Input: part model. Units: mm. Frame: model coordinates. A direction names the side the tool comes from. Round coordinates to 2 decimals unless told otherwise and drop trailing zeros. Order: outer loops, then holes, each group sorted by start corner. A loop starts at its lowest first (then second) coordinate and runs counter-clockwise, first axis right, second up. Notation, with made-up numbers: (65, -15) -> (104, -15) arc R20 cw to (104, -3) -> close; hole circle Ø10 at (-20, -9). An arc over 180 degrees is marked (long way). Answer as CSV lines item,"result". Start each with the question number.
1) Line query: L1, parallel to X at y = -3.75, z = 5.05; L2, parallel to Y at x = 6, z = 2.6; L3, parallel to X at y = 4, z = 2.95. Output: solid intervals per line, ascending.
2) Section query A-A, the plane z = 3.7. Output: boundary loops of the cut face in (x, y), and give its area (3 significant figures).
3) First-contact query: P1, Ø1.8, axis at x = 10, y = -5, coming from the +Z side; P2, Ø0.8, axis at x = 16, y = -3, coming from the +Z side; P3, Ø3, axis at x = 6.5, y = 2.5, coming from the +Z side. Flat tips, straight axial feed; report the tip coordinate or a pass-through.
4) Access query for faces 1 (the face through (1, -5, 5.3)), 2 (the face through (0.5, 1.9, 1.9)), 3 (the face through (16, 3.95, 5)), 4 (the face through (8, 4.25, 4)), 5 (the face through (0.5, 3.95, 4.5)). Directions: +Z, -Z, +X, -X, +Y, -Y. A direction counts if a zero-diameter tool reaches every point of the face in a straight line with its end or side. Return the directions, or none.
5) Section query C-C, the plane y = -1.5. Output: boundary loops of the cut face in (x, z), and give its area (3 significant figures).
6) Section query D-D, the plane z = 2.6. Output: boundary loops of the cut face in (x, y).
7) Mould query, pull axis X, two halves, no side actions, for faces 6 (the face through (2, 0, 4)), 7 (the face through (16.5, 4.3, 2.9)), 8 (the face through (16, 3, 2.9)). Classes: +X half, -X half, draft (parallel to the pull), parting line (faces both ways), or undercut.
8) Section query B-B, the plane x = 2.8. Output: boundary loops of the cut face in (y, z), and give its area (3 significant figures).
```python
from build123d import *

# Parameters (mm, degrees)
BOX019_W          = 12.3
BOX019_H          = 9.7
BOX019_DEPTH      = 1
CYLINDER004_R     = 0.8
CYLINDER004_DEPTH = 20
BOX018_W          = 1.6
BOX018_H          = 20
BOX018_DEPTH      = 3
BOX017_W          = 12.4
BOX017_H          = 8.5
BOX017_DEPTH      = 4.3
BOX013_W          = 1
BOX013_H          = 2.05
BOX013_DEPTH      = 3.3
BOX014_W          = 1
BOX014_H          = 2.05
BOX014_DEPTH      = 3.3
BOX011_W          = 1
BOX011_H          = 2.05
BOX011_DEPTH      = 3.3
BOX012_W          = 1
BOX012_H          = 2.05
BOX012_DEPTH      = 3.3
BOX010_W          = 1
BOX010_H          = 3.8
BOX010_DEPTH      = 5.3
BOX009_W          = 1
BOX009_H          = 3.8
BOX009_DEPTH      = 5.3
BOX007_W          = 16.5
BOX007_H          = 1.05
BOX007_DEPTH      = 1
BOX008_W          = 16.5
BOX008_H          = 1.05
BOX008_DEPTH      = 1
BOX_W             = 16.5
BOX_H             = 11.8
BOX_DEPTH         = 5.3


with BuildPart() as cube016:
    # Box019 → Box019 (new body)
    with BuildSketch(Plane(origin=(2.1, -4.85, 5.3), x_dir=(1, 0, 0), z_dir=(0, 0, 1))):
        with Locations((6.15, 4.85)):
            Rectangle(BOX019_W, BOX019_H)
    extrude(amount=BOX019_DEPTH)


with BuildPart() as cylinder004:
    # Cylinder004 → Cylinder004 (new body)
    with BuildSketch(Plane(origin=(2.8, 10, 5), x_dir=(1, 0, 0), z_dir=(0, -1, 0))):
        Circle(CYLINDER004_R)
    extrude(amount=CYLINDER004_DEPTH)


with BuildPart() as fusion005:
    # Box018 → Box018 (new body)
    with BuildSketch(Plane(origin=(2, -10, 5), x_dir=(1, 0, 0), z_dir=(0, 0, 1))):
        with Locations((0.8, 10)):
            Rectangle(BOX018_W, BOX018_H)
    extrude(amount=BOX018_DEPTH)

    # Fusion005: union Cylinder004
    add(cylinder004.part)


with BuildPart() as cube:
    # Box017 → Box017 (new body)
    with BuildSketch(Plane(origin=(2, -4.25, 1.9), x_dir=(1, 0, 0), z_dir=(0, 0, 1))):
        with Locations((6.2, 4.25)):
            Rectangle(BOX017_W, BOX017_H)
    extrude(amount=BOX017_DEPTH)


with BuildPart() as cube011:
    # Box013 → Box013 (new body)
    with BuildSketch(Plane(origin=(0, 1.9, 2.9), x_dir=(1, 0, 0), z_dir=(0, 0, 1))):
        with Locations((0.5, 1.025)):
            Rectangle(BOX013_W, BOX013_H)
    extrude(amount=BOX013_DEPTH)


with BuildPart() as cube012:
    # Box014 → Box014 (new body)
    with BuildSketch(Plane(origin=(0, -3.95, 2.9), x_dir=(1, 0, 0), z_dir=(0, 0, 1))):
        with Locations((0.5, 1.025)):
            Rectangle(BOX014_W, BOX014_H)
    extrude(amount=BOX014_DEPTH)


with BuildPart() as cube009:
    # Box011 → Box011 (new body)
    with BuildSketch(Plane(origin=(15.5, -3.95, 2.9), x_dir=(1, 0, 0), z_dir=(0, 0, 1))):
        with Locations((0.5, 1.025)):
            Rectangle(BOX011_W, BOX011_H)
    extrude(amount=BOX011_DEPTH)


with BuildPart() as cube010:
    # Box012 → Box012 (new body)
    with BuildSketch(Plane(origin=(15.5, 1.9, 2.9), x_dir=(1, 0, 0), z_dir=(0, 0, 1))):
        with Locations((0.5, 1.025)):
            Rectangle(BOX012_W, BOX012_H)
    extrude(amount=BOX012_DEPTH)


with BuildPart() as cube008:
    # Box010 → Box010 (new body)
    with BuildSketch(Plane(origin=(15.5, -1.9, 0.9), x_dir=(1, 0, 0), z_dir=(0, 0, 1))):
        with Locations((0.5, 1.9)):
            Rectangle(BOX010_W, BOX010_H)
    extrude(amount=BOX010_DEPTH)


with BuildPart() as fusion003:
    # Box009 → Box009 (new body)
    with BuildSketch(Plane(origin=(0, -1.9, 0.9), x_dir=(1, 0, 0), z_dir=(0, 0, 1))):
        with Locations((0.5, 1.9)):
            Rectangle(BOX009_W, BOX009_H)
    extrude(amount=BOX009_DEPTH)

    # Fusion003: union Cube011, Cube012, Cube009, Cube010, Cube008
    add(cube011.part)
    add(cube012.part)
    add(cube009.part)
    add(cube010.part)
    add(cube008.part)


with BuildPart() as cube005:
    # Box007 → Box007 (new body)
    with BuildSketch(Plane(origin=(0, 4.85, 5.3), x_dir=(1, 0, 0), z_dir=(0, 0, 1))):
        with Locations((8.25, 0.525)):
            Rectangle(BOX007_W, BOX007_H)
    extrude(amount=BOX007_DEPTH)


with BuildPart() as fusion002:
    # Box008 → Box008 (new body)
    with BuildSketch(Plane(origin=(0, -5.9, 5.3), x_dir=(1, 0, 0), z_dir=(0, 0, 1))):
        with Locations((8.25, 0.525)):
            Rectangle(BOX008_W, BOX008_H)
    extrude(amount=BOX008_DEPTH)

    # Fusion002: union Cube005
    add(cube005.part)


with BuildPart() as cut006:
    # Box → Box (new body)
    with BuildSketch(Plane(origin=(0, -5.9, 0.9), x_dir=(1, 0, 0), z_dir=(0, 0, 1))):
        with Locations((8.25, 5.9)):
            Rectangle(BOX_W, BOX_H)
    extrude(amount=BOX_DEPTH)

    # Cut002: cut Fusion002
    add(fusion002.part, mode=Mode.SUBTRACT)

    # Cut003: cut Fusion003
    add(fusion003.part, mode=Mode.SUBTRACT)

    # Cut004: cut Cube
    add(cube.part, mode=Mode.SUBTRACT)

    # Cut005: cut Fusion005
    add(fusion005.part, mode=Mode.SUBTRACT)

    # Cut006: cut Cube016
    add(cube016.part, mode=Mode.SUBTRACT)


solid = cut006.part
```
Findings:
1,L1,"x = 1 to 2, 14.4 to 15.5"
1,L2,"y = -5.9 to -4.25, 4.25 to 5.9"
1,L3,"x = 0 to 2, 14.4 to 16.5"
2,outline,"(0, -5.9) -> (16.5, -5.9) -> (16.5, -3.95) -> (15.5, -3.95) -> (15.5, 3.95) -> (16.5, 3.95) -> (16.5, 5.9) -> (0, 5.9) -> (0, 3.95) -> (1, 3.95) -> (1, -3.95) -> (0, -3.95) -> close; hole (2, -4.25) -> (14.4, -4.25) -> (14.4, 4.25) -> (2, 4.25) -> close"
2,area,"73.5 mm^2"
3,P1,"stops at z = 5.3"
3,P2,"stops at z = 2.9"
3,P3,"stops at z = 1.9"
4,face 1,"+Z, +X, -X, -Y"
4,face 2,"+Z, -Z, -X"
4,face 3,"+Z, +X"
4,face 4,"+Z"
4,face 5,"+Z, -X"
5,outline,"(1, 0.9) -> (15.5, 0.9) -> (15.5, 6.2) -> (14.4, 6.2) -> (14.4, 1.9) -> (2, 1.9) -> (2, 6.2) -> (1, 6.2) -> close"
5,area,"23.5 mm^2"
6,outline,"(0, -5.9) -> (16.5, -5.9) -> (16.5, -1.9) -> (15.5, -1.9) -> (15.5, 1.9) -> (16.5, 1.9) -> (16.5, 5.9) -> (0, 5.9) -> (0, 1.9) -> (1, 1.9) -> (1, -1.9) -> (0, -1.9) -> close; hole (2, -4.25) -> (14.4, -4.25) -> (14.4, 4.25) -> (2, 4.25) -> close"
7,face 6,"undercut"
7,face 7,"+X half"
7,face 8,"draft"
8,outline,"(-5.9, 0.9) -> (5.9, 0.9) -> (5.9, 4.2) -> (4.25, 4.2) -> (4.25, 1.9) -> (-4.25, 1.9) -> (-4.25, 4.2) -> (-5.9, 4.2) -> close"
8,area,"19.4 mm^2"
